```python
from build123d import *

# Parameters (mm, degrees)
F0_R     = 6.179709
F1_DEPTH = 12.7


with BuildPart() as f1:
    # F0 (on Top) → F1 (new body)
    with BuildSketch(Plane.XY):
        Polygon((6.35, -6.35), (23.169448, 0), (23.514125, 0.130129), (6.35, 6.35), (0, 25.4), (-6.35, 6.35), (-25.4, 0), (-6.35, -6.35), (0, -25.4), align=None)
        Circle(F0_R, mode=Mode.SUBTRACT)
    extrude(amount=F1_DEPTH)


solid = f1.part
```
Source: CAD feature listing. Evaluate the final solid. Frame: model axes, mm. Give positions to 0.01 mm unless a question says otherwise; leave off trailing zeros. Write each loop counter-clockwise with the first axis right and the second up, starting at its lowest first coordinate (ties: lowest second). Pieces come first, ordered by that corner, then holes. Notation, with made-up numbers: (48.25, 4) - (81.25, 4) arc R28 cw to (81.25, 39) - close; hole circle Ø4 at (-11.75, 55). An arc over 180 degrees is marked (long way). One line per item, written item: value. Start each with the question number.
Q1. Material intervals for probe 1 along X at (y, z) = (7.5, 1.25); probe 2 along X at (y, z) = (-8, 1); probe 3 along Y at (x, z) = (-22, 3.25), sorted ascending. Write a range as from..to.
Q2. Section query D-D, the plane y = -21.5. Return the cut outline in (x, z), then the cut area to 3 significant figures.
Q3. Section query A-A, the plane y = -2. Return the cut outline in (x, z).
Q4. Section query C-C, the plane x = -5. Return the cut outline in (y, z), then the cut area to 3 significant figures.
Q5. Section query B-B, the plane z = 11.75. Return the cut outline in (x, y).
Q6. First-contact query: pin 1 Ø4 at (x, y) = (-14.5, -5.5) entering from +Z; pin 2 Ø1.5 at (y, z) = (7.5, 9) entering from -X; pin 3 Ø5 at (x, z) = (-15.5, 9) entering from +Y; pin 4 Ø1.5 at (x, z) = (-19.5, 8) entering from -Y. Flat tips, straight axial feed; report the tip coordinate or a pass-through.
Q7. Draft query along Y for faces 1 (the face through (-6.174, 0.272, 6.261)), 2 (the face through (-6.5, 0.1, 12.7)), 3 (the face through (-15.74, 3.22, 6.26)). Return one class per face: +Y half, -Y half, draft (parallel to the pull), parting line (faces both ways), or undercut.
Answer:
1. probe 1: x = -5.97..5.97
1. probe 2: x = -5.8..5.8
1. probe 3: y = -1.13..1.13
2. outline: (-1.3, 0) - (1.3, 0) - (1.3, 12.7) - (-1.3, 12.7) - close
2. area: 33.0 mm2
3. outline: (-19.4, 0) - (-5.85, 0) - (-5.85, 12.7) - (-19.4, 12.7) - close; (5.85, 0) - (17.87, 0) - (17.87, 12.7) - (5.85, 12.7) - close
4. outline: (-10.4, 0) - (-3.63, 0) - (-3.63, 12.7) - (-10.4, 12.7) - close; (3.63, 0) - (10.4, 0) - (10.4, 12.7) - (3.63, 12.7) - close
4. area: 172 mm2
5. outline: (-25.4, 0) - (-6.35, -6.35) - (0, -25.4) - (6.35, -6.35) - (23.17, 0) - (23.51, 0.13) - (6.35, 6.35) - (0, 25.4) - (-6.35, 6.35) - close; hole circle Ø12.36 at (0, 0)
6. pin 1: stops at z = 12.7
6. pin 2: stops at x = -6.22
6. pin 3: stops at y = 4.13
6. pin 4: stops at y = -2.22
7. face 1: undercut
7. face 2: draft
7. face 3: +Y half
